Can you work these out from the model? Positions are in its coordinate system, mm. Face numbers are marked on the shaded views. A direction names the side the tool comes from. Round coordinates to 2 decimals unless told otherwise and drop trailing zeros. Order: outer loops, then holes, each group sorted by start corner. A loop starts at its lowest first (then second) coordinate and runs counter-clockwise, first axis right, second up. Notation, with made-up numbers: (-2.5, 34) -> (56.5, 34) arc R24 ccw to (56.5, 45) -> close; hole circle Ø8 at (84.5, 41). An arc over 180 degrees is marked (long way). Use a Markdown table: item, result. Add a question column.
Q1. If we section it at B-B on z = 1335: List the corners of the cut face in (x, y) for me, plus the area to 3 significant figures.
Q2. If we section it at A-A on x = -1601: List the corners of the cut face in (y, z) for me.
Q3. I'm going to push flat-ended pins straight in: pin 1 Ø8 at (x, y) = (-1596.5, 759) entering from -Z; pin 2 Ø4.5 at (y, z) = (759.85, 1339.83) entering from +X; pin 3 Ø3 at (x, z) = (-1633.5, 1243) entering from -Y. Where does each tip first touch, or does it pass through?
Q4. For the marked faces 1 and 2, which set-ups out of +Z, -Z, +X, -X, +Y, -Y let a thin tool reach every point of the face, with its end or its side?
Q5. I need wall thicknesses on line 1 along Y through (x, z) = (-1555, 1213); line 2 along Z through (x, y) = (-1558.5, 754.75); line 3 along X through (y, z) = (755, 1336). Which ranges of each line are inside material? Lowest first, please. Write a range as [from, to].
```python
from build123d import *

# Parameters (mm, degrees)
SKETCH1_W           = 180
SKETCH1_H           = 18
SKETCH1_R           = 1.7
BOSS_EXTRUDE1_DEPTH = 4
SKETCH2_W           = 100
SKETCH2_H           = 18
SKETCH2_R           = 1.7
BOSS_EXTRUDE2_DEPTH = 4
SKETCH3_W           = 96
SKETCH3_H           = 4
BOSS_EXTRUDE3_DEPTH = 176


with BuildPart() as part:
    # Sketch1 → Boss-Extrude1 (new body)
    with BuildSketch(Plane(origin=(-1647.169528543, 0, 0), x_dir=(0, 0, -1), z_dir=(1, 0, 0))):
        with Locations((-1279.825666692, 760.849345995)):
            Rectangle(SKETCH1_W, SKETCH1_H)
        with Locations((-1219.825666692, 759.849345995)):
            Circle(SKETCH1_R, mode=Mode.SUBTRACT)
        with Locations((-1339.825666692, 759.849345995)):
            Circle(SKETCH1_R, mode=Mode.SUBTRACT)
    extrude(amount=BOSS_EXTRUDE1_DEPTH)

    # Sketch2 → Boss-Extrude2 (add)
    with BuildSketch(Plane(origin=(0, 0, 1369.825666692), x_dir=(-1, 0, 0), z_dir=(0, 0, -1))):
        with Locations((1597.169528543, 760.849345995)):
            Rectangle(SKETCH2_W, SKETCH2_H)
        with Locations((1617.169528543, 759.849345995)):
            Circle(SKETCH2_R, mode=Mode.SUBTRACT)
        with Locations((1562.169528543, 759.849345995)):
            Circle(SKETCH2_R, mode=Mode.SUBTRACT)
    extrude(amount=BOSS_EXTRUDE2_DEPTH)

    # Sketch3 → Boss-Extrude3 (add)
    with BuildSketch(Plane(origin=(0, 0, 1365.825666692), x_dir=(-1, 0, 0), z_dir=(0, 0, -1))):
        with Locations((1595.169528543, 767.849345995)):
            Rectangle(SKETCH3_W, SKETCH3_H)
    extrude(amount=BOSS_EXTRUDE3_DEPTH)


solid = part.part
```
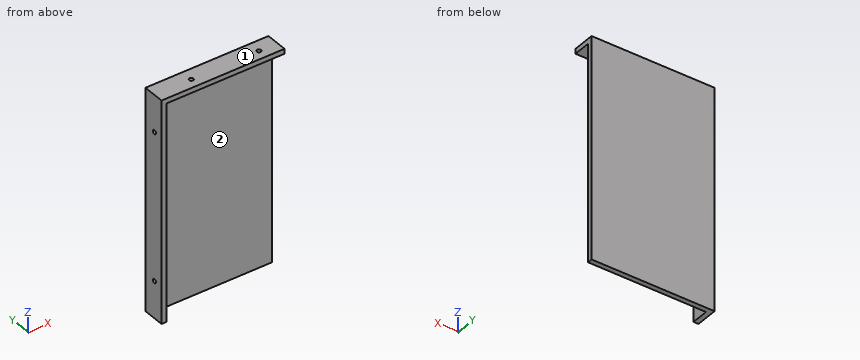
Answer below:
| question | item | result |
|---|---|---|
| 1 | outline | (-1647.17, 751.85) -> (-1643.17, 751.85) -> (-1643.17, 765.85) -> (-1547.17, 765.85) -> (-1547.17, 769.85) -> (-1647.17, 769.85) -> close |
| 1 | area | 456 mm² |
| 2 | outline | (751.85, 1365.83) -> (765.85, 1365.83) -> (765.85, 1189.83) -> (769.85, 1189.83) -> (769.85, 1369.83) -> (751.85, 1369.83) -> close |
| 3 | pin 1 | z = 1365.83 |
| 3 | pin 2 | x = -1643.17 |
| 3 | pin 3 | y = 765.85 |
| 4 | face 1 | +Z, +X, -X, +Y, -Y |
| 4 | face 2 | -Z, +X, -Y |
| 5 | line 1 | [765.85, 769.85] |
| 5 | line 2 | [1365.83, 1369.83] |
| 5 | line 3 | [-1647.17, -1643.17] |
